Read the model definition and answer for the solid it produces. Units are mm, in the model's axes. A direction names the side the tool comes from. Round coordinates to 2 decimals unless told otherwise and drop trailing zeros. Order: outer loops, then holes, each group sorted by start corner. A loop starts at its lowest first (then second) coordinate and runs counter-clockwise, first axis right, second up. Notation, with made-up numbers: (-25.5, 35.5) - (-20.5, 35.5) arc R21 cw to (-20.5, 71.5) - close; hole circle Ø6 at (63.5, 57). An arc over 180 degrees is marked (long way). Put each result on its own line as item: value. Start each with the question number.
Q1. Section C-C on x = 48 is taken. Give the vertices of the cut face in (y, z) (3 decimals).
Q2. Each of these flat-tipped pins is pushed along its axis until it touches: pin 1 Ø3 at (x, y) = (24, 13) entering from -Z; pin 2 Ø6 at (x, z) = (31, 20) entering from +Y; pin 3 Ø19 at (x, y) = (82.55, 82.55) entering from +Z (3 decimals); pin 4 Ø2 at (x, z) = (60.5, 21.5) entering from +Y. Where does it stop, or does it pass through?
Q3. Section D-D on z = 3 is taken. Give the vertices of the cut face in (x, y) (3 decimals), then the cut area to 3 significant figures.
Q4. Section A-A on y = 12.7 is taken. Give the vertices of the cut face in (x, z) (3 decimals).
Q5. Find the intervals of material crossed by line 1 along X through (y, z) = (82.55, 5.5); line 2 along Y through (x, z) = (7.5, 14.5), in increasing order. Write a range as from..to.
Q6. For a pull along X with two mould halves and no side action, classify faces 1 (the face through (48, 95.25, 8)), 2 (the face through (9.95, 17.98, 8.05)), 3 (the face through (31.8, 41.1, 25.7)), 4 (the face through (0, 48, 8)) as pulls with the +X half, pulls with the -X half, needs draft (parallel to the pull), parting line crosses it, or undercut.
Q7. Which of the six approach directions +Z, -Z, +X, -X, +Y, -Y give full straight-line access (tool end or side, diameter ignored) to faces 5 (the face through (35.5, 51.4, 17.6)), 6 (the face through (47, 69, 15.875))?
Autodesk Fusion 360 part; units mm, degrees
sketch "Sketch4" plane through (0, 0, 0) normal (0, 0, 1) x (1, 0, 0)
  line L0 (0, 0) -> (95.25, 0)
  line L1 (95.25, 0) -> (95.25, 95.25)
  line L2 (95.25, 95.25) -> (0, 95.25)
  line L3 (0, 95.25) -> (0, 0)
  dimension "d17" = 95.25
  dimension "d18" = 95.25
extrude "Extrude4" add sketch "Sketch4" along normal blind 15.875
sketch "Sketch5" plane through (0, 0, 15.875) normal (0, 0, 1) x (-1, 0, 0)
  line L0 (0, -95.25) -> (0, 0)
  line L1 (0, 0) -> (-95.25, 0)
  line L2 (-95.25, 0) -> (-95.25, -95.25)
  line L3 (-95.25, -95.25) -> (0, -95.25)
  line L4 (0, -95.25) -> (-47.625, -95.25)
  line L5 (-47.625, -95.25) -> (-47.625, -47.625)
  line L6 (-47.625, -47.625) -> (0, -47.625)
  line L7 (0, -47.625) -> (0, -95.25)
  circle A0 centre (-47.625, -47.625) radius 12.7
  dimension "d21" = 47.625
  dimension "d22" = 47.625
  dimension "d23" = 25.4
extrude "Extrude5" cut sketch "Sketch5" against normal blind 25 contours L5 L6 A0 | L5 L6 A0
sketch "Sketch6" plane through (0, 0, 15.875) normal (0, 0, 1) x (-1, 0, 0)
  circle A0 centre (-47.625, -47.625) radius 12.7
  line L0 (0, -95.25) -> (0, 0)
  line L1 (0, 0) -> (-95.25, 0)
  line L2 (-95.25, 0) -> (-95.25, -95.25)
  line L3 (-95.25, -95.25) -> (0, -95.25)
  circle A1 centre (-47.625, -47.625) radius 17.1179
extrude "Extrude6" add sketch "Sketch6" along normal blind 19.8438 contours A1
sketch "Sketch7" plane through (0, 0, 15.875) normal (0, 0, 1) x (-1, 0, 0)
  circle A0 centre (-47.625, -47.625) radius 17.1179
  line L0 (0, -95.25) -> (0, 0)
  line L1 (0, 0) -> (-95.25, 0)
  line L2 (-95.25, 0) -> (-95.25, -95.25)
  line L3 (-95.25, -95.25) -> (0, -95.25)
  circle A1 centre (-47.625, -47.625) radius 34.925
  line L4 (-47.625, -95.25) -> (-47.625, -82.55)
  line L5 (0, -50) -> (-12.7808, -50)
  line L6 (0, -95.25) -> (-12.7, -95.25)
  line L7 (-12.7, -95.25) -> (-12.7, -82.55)
  line L8 (-12.7, -82.55) -> (0, -82.55)
  line L9 (0, -82.55) -> (0, -95.25)
  line L10 (-95.25, -95.25) -> (-82.55, -95.25)
  line L11 (-82.55, -95.25) -> (-82.55, -82.55)
  line L12 (-82.55, -82.55) -> (-95.25, -82.55)
  line L13 (-95.25, -82.55) -> (-95.25, -95.25)
  line L14 (0, 0) -> (-12.7, 0)
  line L15 (-12.7, 0) -> (-12.7, -12.7)
  line L16 (-12.7, -12.7) -> (0, -12.7)
  line L17 (0, -12.7) -> (0, 0)
  line L18 (-95.25, 0) -> (-82.55, 0)
  line L19 (-82.55, 0) -> (-82.55, -12.7)
  line L20 (-82.55, -12.7) -> (-95.25, -12.7)
  line L21 (-95.25, -12.7) -> (-95.25, 0)
  circle A2 centre (-12.7, -82.55) radius 4.7625
  circle A3 centre (-82.55, -82.55) radius 4.7625
  circle A4 centre (-12.7, -12.7) radius 4.7625
  circle A5 centre (-82.55, -12.7) radius 4.7625
  dimension "d28" = 69.85
  dimension "d29" = 12.7
  dimension "d30" = 12.7
  dimension "d31" = 12.7
  dimension "d32" = 12.7
  dimension "d33" = 12.7
  dimension "d34" = 12.7
  dimension "d35" = 12.7
  dimension "d36" = 12.7
  dimension "d37" = 9.525
  dimension "d38" = 9.525
  dimension "d39" = 9.525
  dimension "d40" = 9.525
extrude "Extrude7" cut sketch "Sketch7" against normal blind 30 contours L7 L8 A2 | L7 L8 A2 | L15 L16 A4 | L15 L16 A4 | L11 L12 A3 | L11 L12 A3 | L19 L20 A5 | L19 L20 A5
sketch "Sketch8" plane through (0, 0, 15.875) normal (0, 0, 1) x (-1, 0, 0)
  circle A0 centre (-12.7, -12.7) radius 4.7625
  circle A1 centre (-82.55, -12.7) radius 4.7625
  circle A2 centre (-12.7, -82.55) radius 4.7625
  circle A3 centre (-82.55, -82.55) radius 4.7625
  circle A4 centre (-47.625, -47.625) radius 17.1179
  line L0 (0, -95.25) -> (0, 0)
  line L1 (0, 0) -> (-95.25, 0)
  line L2 (-95.25, 0) -> (-95.25, -95.25)
  line L3 (-95.25, -95.25) -> (0, -95.25)
  circle A5 centre (-12.7, -12.7) radius 5.953
  circle A6 centre (-12.7, -82.55) radius 5.953
  circle A7 centre (-82.55, -82.55) radius 5.953
  circle A8 centre (-82.55, -12.7) radius 5.953
  dimension "d43" = 11.906
  dimension "d44" = 11.906
  dimension "d45" = 11.906
  dimension "d46" = 11.906
extrude "Extrude8" cut sketch "Sketch8" against normal blind 35 contours A5 | A6 | A7 | A8
equation "d21 = ( 95.25 / 2 ) * 1 mm"
equation "d22 = ( 95.25 / 2 ) * 1 mm"
equation "d23 = ( 12.7 * 2 ) * 1 mm"
Findings:
1. outline: (0, 0) - (34.931, 0) - (34.931, 35.719) - (30.511, 35.719) - (30.511, 15.875) - (0, 15.875) - close; (60.319, 0) - (95.25, 0) - (95.25, 15.875) - (64.739, 15.875) - (64.739, 35.719) - (60.319, 35.719) - close
2. pin 1: z = 0
2. pin 2: y = 57.99
2. pin 3: z = 15.875
2. pin 4: y = 59.95
3. outline: (0, 0) - (95.25, 0) - (95.25, 95.25) - (0, 95.25) - close; hole circle Ø11.906 at (12.7, 12.7); hole circle Ø11.906 at (12.7, 82.55); hole circle Ø25.4 at (47.625, 47.625); hole circle Ø11.906 at (82.55, 12.7); hole circle Ø11.906 at (82.55, 82.55)
3. area: 8,120 mm2
4. outline: (0, 0) - (6.747, 0) - (6.747, 15.875) - (0, 15.875) - close; (18.653, 0) - (76.597, 0) - (76.597, 15.875) - (18.653, 15.875) - close; (88.503, 0) - (95.25, 0) - (95.25, 15.875) - (88.503, 15.875) - close
5. line 1: 0..6.75, 18.65..76.6, 88.5..95.25
5. line 2: 0..9.8, 15.6..79.65, 85.45..95.25
6. face 1: needs draft
6. face 2: undercut
6. face 3: parting line crosses it
6. face 4: pulls with the -X half
7. face 5: +Z, -Z
7. face 6: +Z
